The drawing under review shows one solid part. Ordinate dimensions are in mm from its lowest x, y, z. A direction names the side the tool comes from. Give positions to 0.01 mm unless a question says otherwise; leave off trailing zeros. Loops run counter-clockwise (first coordinate to the right, second up) from the corner with the lowest first, then second, coordinate; pieces in that order, holes last. Notation, with made-up numbers: (81.25, 25.25) -> (123.25, 25.25) arc R25 cw to (123.25, 46.25) -> close; hole circle Ø2 at (-27, 85). An arc over 180 degrees is marked (long way). Answer in a Markdown table with one row per item. Add a question column.
(1) Draft analysis for pull direction X (two halves, no side actions). For the marked faces 6, 7 and 8, state which applies: +X half, -X half, draft (parallel to the pull), parting line (faces both ways), or undercut.
(2) For pin 1 (6 mm diameter, centred on y = 11.5, z = 4, fed in from -X); pin 2 (1 mm diameter, centred on x = 59, y = 16, fed in from -Z); pin 3 (5 mm diameter, centred on x = 5, z = 5, fed in from +Y), all flat-tipped, find the tip position at first contact; note any pin that passes through.
(3) Consider section D-D on z = 4.25. Write out the cut boundary in (x, y), then the cut area to 3 significant figures.
(4) Consider section C-C on x = 51. Write out the cut boundary in (y, z).
(5) For line 1 (X direction, y = 30, z = 19.05); line 2 (X direction, y = 6, z = 10.75); line 3 (Y direction, x = 36, z = 19.05), list the stretches that pass through material, from the lowest coordinate up.
(6) Consider section A-A on x = 30. Write out the cut boundary in (y, z), then the cut area to 3 significant figures.
(7) Consider section B-B on y = 30. Write out the cut boundary in (x, z), then the cut area to 3 significant figures.
(8) For the marked faces 1, 2, 3, 4 and 5, list the 3-axis set-ups (+Z, -Z, +X, -X, +Y, -Y) from which the entire face can be reached by the end or side of a thin tool; tool diameter is ignored.
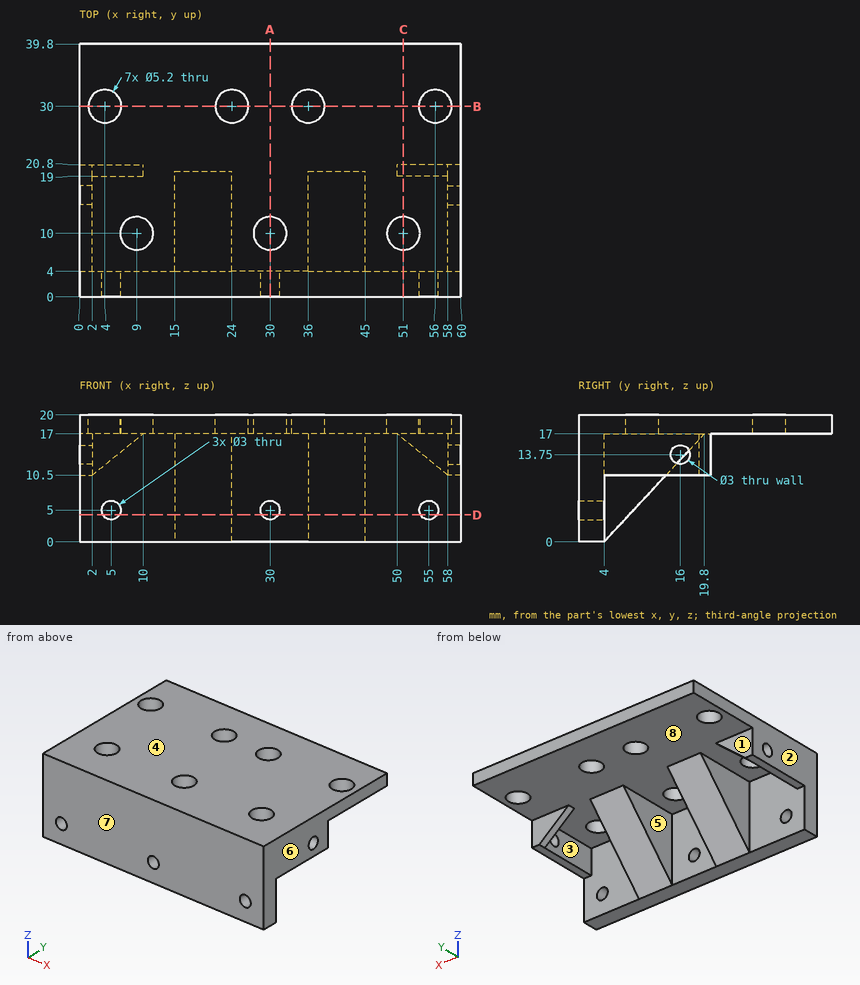
Values follow:
| question | item | result |
|---|---|---|
| 1 | face 6 | +X half |
| 1 | face 7 | draft |
| 1 | face 8 | undercut |
| 2 | pin 1 | x = 15 |
| 2 | pin 2 | z = 10.5 |
| 2 | pin 3 | y = 4 |
| 3 | outline | (0, 0) -> (3.7, 0) -> (3.7, 4) -> (0, 4) -> close; (6.3, 0) -> (28.7, 0) -> (28.7, 4) -> (24, 4) -> (24, 7.95) -> (15, 7.95) -> (15, 4) -> (6.3, 4) -> close; (31.3, 0) -> (53.7, 0) -> (53.7, 4) -> (45, 4) -> (45, 7.95) -> (36, 7.95) -> (36, 4) -> (31.3, 4) -> close; (56.3, 0) -> (60, 0) -> (60, 4) -> (56.3, 4) -> close |
| 3 | area | 280 mm2 |
| 4 | outline | (0, 0) -> (4, 0) -> (4, 17) -> (7.4, 17) -> (7.4, 20) -> (0, 20) -> close; (12.6, 17) -> (19, 17) -> (19, 16.19) -> (20.8, 16.19) -> (20.8, 17) -> (39.8, 17) -> (39.8, 20) -> (12.6, 20) -> close |
| 5 | line 1 | 0 to 1.4, 6.6 to 21.4, 26.6 to 33.4, 38.6 to 53.4, 58.6 to 60 |
| 5 | line 2 | 0 to 2, 15 to 24, 36 to 45, 58 to 60 |
| 5 | line 3 | 0 to 27.4, 32.6 to 39.8 |
| 6 | outline | (0, 0) -> (4, 0) -> (4, 3.5) -> (0, 3.5) -> close; (0, 6.5) -> (4, 6.5) -> (4, 17) -> (7.4, 17) -> (7.4, 20) -> (0, 20) -> close; (12.6, 17) -> (39.8, 17) -> (39.8, 20) -> (12.6, 20) -> close |
| 6 | area | 160 mm2 |
| 7 | outline | (0, 17) -> (1.4, 17) -> (1.4, 20) -> (0, 20) -> close; (6.6, 17) -> (21.4, 17) -> (21.4, 20) -> (6.6, 20) -> close; (26.6, 17) -> (33.4, 17) -> (33.4, 20) -> (26.6, 20) -> close; (38.6, 17) -> (53.4, 17) -> (53.4, 20) -> (38.6, 20) -> close; (58.6, 17) -> (60, 17) -> (60, 20) -> (58.6, 20) -> close |
| 7 | area | 118 mm2 |
| 8 | face 1 | -Z, +X, -X, +Y |
| 8 | face 2 | +Z, -Z, -X, +Y, -Y |
| 8 | face 3 | -Z |
| 8 | face 4 | +Z, +X, -X, +Y, -Y |
| 8 | face 5 | -Z, +Y |
